Verification items for the finished model (mm, model axes). A direction names the side the tool comes from. Round coordinates to 2 decimals unless told otherwise and drop trailing zeros. Write each loop counter-clockwise with the first axis right and the second up, starting at its lowest first coordinate (ties: lowest second). Pieces come first, ordered by that corner, then holes. Notation, with made-up numbers: M 78,13.25 L 119,13.25 A17 ccw 119,32.25 Z; hole C 21,-1 d1. An arc over 180 degrees is marked long. Write each question's results on one line, items separated by ' | '.
from build123d import *

# Parameters (mm, degrees)
SKETCH1_R           = 9.525
BOSS_EXTRUDE1_DEPTH = 25.4
SKETCH2_R           = 3.175
CUT_EXTRUDE1_DEPTH  = 12.7
SKETCH4_R           = 1.5875
CUT_EXTRUDE2_DEPTH  = 29.750847814
SKETCH5_R           = 3.01625
CUT_EXTRUDE3_DEPTH  = 19.513272438


with BuildPart() as part:
    # Sketch1 → Boss-Extrude1 (new body)
    with BuildSketch(Plane(origin=(0, 0, 0), x_dir=(1, 0, 0), z_dir=(0, 1, 0))):
        with Locations(Location((0, 0, 0), (0, 0, 270))):
            Circle(SKETCH1_R)
    extrude(amount=BOSS_EXTRUDE1_DEPTH)

    # Sketch2 → Cut-Extrude1 (cut)
    with BuildSketch(Plane(origin=(0, 25.4, 0), x_dir=(1, 0, 0), z_dir=(0, 1, 0))):
        with Locations(Location((0, 0, 0), (0, 0, 270))):
            Circle(SKETCH2_R)
    extrude(amount=-CUT_EXTRUDE1_DEPTH, mode=Mode.SUBTRACT)

    # Sketch4 → Cut-Extrude2 (cut, through all)
    with BuildSketch(Plane.XY):
        with Locations(Location((0, 22.225, 0), (0, 0, 270))):
            Circle(SKETCH4_R)
        with Locations(Location((0, 3.175, 0), (0, 0, 90))):
            Circle(SKETCH4_R)
    extrude(amount=CUT_EXTRUDE2_DEPTH, mode=Mode.SUBTRACT)

    # Sketch5 → Cut-Extrude3 (cut, through all)
    with BuildSketch(Plane(origin=(0, 12.7, 0), x_dir=(1, 0, 0), z_dir=(0, 1, 0))):
        with Locations(Location((0, 0, 0), (0, 0, 270))):
            Circle(SKETCH5_R)
    extrude(amount=-CUT_EXTRUDE3_DEPTH, mode=Mode.SUBTRACT)


solid = part.part
1) Access from +Z, -Z, +X, -X, +Y, -Y to the whole of each face (thin tool, end or side, straight path). Record for faces 1 (the flat face through (0, 25.4, 4)), 2 (the cylindrical face through (0.14, 19.14, -3.17)), 3 (the cylindrical face through (-0.07, 1.59, 6)).
Calculated:
face 1: +Z, -Z, +X, -X, +Y | face 2: +Y | face 3: +Z
2) Depth check by flat-ended pin: P1, Ø2, axis at x = -2.5, y = 22.5, coming from the +Z side; P2, Ø4, axis at x = -6, y = 11.5, coming from the -Z side; P3, Ø5, axis at y = 9, z = 3, coming from the -X side. Enter the tip coordinate at first touch or a pass-through.
Calculated:
P1: stops at z = 9.4 | P2: stops at z = -8.64 | P3: stops at x = -9.51
3) Sectioned sample at B-B, the plane z = 0. Record the cut outline in (x, y) (3 decimals).
Calculated:
outline: M -9.525,0 L -3.016,0 L -3.016,12.7 L -3.175,12.7 L -3.175,25.4 L -9.525,25.4 Z; M 3.016,0 L 9.525,0 L 9.525,25.4 L 3.175,25.4 L 3.175,12.7 L 3.016,12.7 Z
4) Draft check along X on faces 4 (the cylindrical face through (-5.796, 12.522, -7.559)), 5 (the cylindrical face through (0.133, 6.439, -3.013)), 6 (the flat face through (2.3, 0, -2.3)). Enter one of: pulls with the +X half, pulls with the -X half, needs draft (parallel to the pull), parting line crosses it, or undercut.
Calculated:
face 4: parting line crosses it | face 5: undercut | face 6: needs draft
5) Sectioned sample at C-C, the plane y = 13.75. Record the cut outline in (x, z) (3 decimals).
Calculated:
outline: C 0,0 d19.05; hole C 0,0 d6.35
6) Material ranges on line 1 (Y direction, x = 0, z = 5); line 2 (X direction, y = 20.25, z = 0) (3 decimals); line 3 (Y direction, x = -0.25, z = 5.5), recorded low to high. Write a range as [from, to].
Calculated:
line 1: y = [0, 1.59], [4.76, 20.64], [23.81, 25.4] | line 2: x = [-9.525, -3.175], [3.175, 9.525] | line 3: y = [0, 1.61], [4.74, 20.66], [23.79, 25.4]
7) Sectioned sample at A-A, the plane x = 0. Count the separate pieces of the cut face and the enclosed holes in it, and give its area (3 significant figures).
Calculated:
separate pieces: 4 | enclosed holes: 0 | area: 286 mm²
8) Sectioned sample at D-D, the plane z = -2.5. Record the cut outline in (x, y).
Calculated:
outline: M -9.19,0 L -1.69,0 L -1.69,12.7 L -1.96,12.7 L -1.96,25.4 L -9.19,25.4 Z; M 1.69,0 L 9.19,0 L 9.19,25.4 L 1.96,25.4 L 1.96,12.7 L 1.69,12.7 Z
